The listing builds one solid part. Answer for the finished solid, in the listing's coordinates (mm). A direction names the side the tool comes from. Round coordinates to 2 decimals unless told otherwise and drop trailing zeros. Order: outer loops, then holes, each group sorted by start corner. A loop starts at its lowest first (then second) coordinate and runs counter-clockwise, first axis right, second up. Notation, with made-up numbers: (72.25, -32) - (114.25, -32) arc R27 cw to (114.25, -14) - close; hole circle Ø3 at (34.5, 10.5). An arc over 180 degrees is marked (long way). Use CSV: the item, a comma, the result in double quotes. Start each with the question number.
Item 1: Find section D-D, the plane z = -16. Give the vertices of the cut face in (x, y), plus the area to 3 significant figures.
Item 2: Determine the mould class of faces 3 (the flat face through (10.9, 25.04, 7.68)), 4 (the flat face through (-13, 50.8, 4)), 5 (the cylindrical face through (-15.12, 25.04, 11.59)) for opening direction X: +X half, -X half, draft (parallel to the pull), parting line (faces both ways), or undercut.
Item 3: Find section A-A, the plane x = 0. Give the vertices of the cut face in (y, z), plus the area to 3 significant figures.
Item 4: Find section C-C, the plane y = 3. Give the vertices of the cut face in (x, z), plus the area to 3 significant figures.
Item 5: Flat-ended cylindrical pins translate along their axes: P1, Ø8, axis at y = 31, z = 5.5, coming from the -X side; P2, Ø8, axis at x = -5, y = 38.5, coming from the -Z side; P3, Ø8, axis at y = 7, z = 10.5, coming from the +X side. Find the tip coordinate at first contact, or state that the pin passes through.
Item 6: For faces 1 (the flat face through (12.102, 25.044, -5.6)), 2 (the flat face through (-13, 0, 4)), determine the directions among +Z, -Z, +X, -X, +Y, -Y from which every point of the face is accessible in a straight line to the end or side of a thin tool.
Item 7: Find section B-B, the plane z = 0. Give the vertices of the cut face in (x, y), plus the area to 3 significant figures.
Item 8: Straight lines are drawn through the part: line 1 along X through (y, z) = (40, 2.5); line 2 along X through (y, z) = (40, 1.5); line 3 along Z through (x, y) = (2.5, 20). For each, find the intervals that lie inside material, in ascending order. Write a range as [from, to].
```python
from build123d import *

# Parameters (mm, degrees)
SKETCH1_R           = 19.05
BOSS_EXTRUDE1_DEPTH = 50.8
CUT_EXTRUDE1_DEPTH  = 50.8


with BuildPart() as part:
    # Sketch1 → Boss-Extrude1 (new body)
    with BuildSketch(Plane(origin=(0, 0, 0), x_dir=(1, 0, 0), z_dir=(0, 1, 0))):
        Circle(SKETCH1_R)
    extrude(amount=BOSS_EXTRUDE1_DEPTH)

    # Sketch2 → Cut-Extrude1 (cut)
    with BuildSketch(Plane.XZ):
        Polygon((-15.323636661, -1.510781079), (-6.353443536, -14.026049167), (8.970193125, -12.515268087), (15.323636661, 1.510781079), (6.353443536, 14.026049167), (-8.970193125, 12.515268087), align=None)
    extrude(amount=-CUT_EXTRUDE1_DEPTH, mode=Mode.SUBTRACT)


solid = part.part
```
Worked out:
1,outline,"(-10.34, 0) - (10.34, 0) - (10.34, 50.8) - (-10.34, 50.8) - close"
1,area,"1,050 mm²"
2,face 3,"undercut"
2,face 4,"draft"
2,face 5,"parting line"
3,outline,"(0, -19.05) - (50.8, -19.05) - (50.8, -13.4) - (0, -13.4) - close; (0, 13.4) - (50.8, 13.4) - (50.8, 19.05) - (0, 19.05) - close"
3,area,"574 mm²"
4,outline,"circle Ø38.1 at (0, 0); hole (-15.32, -1.51) - (-6.35, -14.03) - (8.97, -12.52) - (15.32, 1.51) - (6.35, 14.03) - (-8.97, 12.52) - close"
4,area,"524 mm²"
5,P1,"stops at x = -18.99"
5,P2,"stops at z = -19.02"
5,P3,"stops at x = 17.91"
6,face 1,"+Y, -Y"
6,face 2,"+Z, -Z, +X, -X, -Y"
7,outline,"(-19.05, 0) - (-14.64, 0) - (-14.64, 50.8) - (-19.05, 50.8) - close; (14.64, 0) - (19.05, 0) - (19.05, 50.8) - (14.64, 50.8) - close"
7,area,"448 mm²"
8,line 1,"x = [-18.89, -13.51], [14.61, 18.89]"
8,line 2,"x = [-18.99, -13.96], [15.32, 18.99]"
8,line 3,"z = [-18.89, -13.15], [13.65, 18.89]"
